```python
from build123d import *

# Parameters (mm, degrees)
SKETCH1_R           = 10
BOSS_EXTRUDE1_DEPTH = 15
CUT_EXTRUDE1_DEPTH  = 16
CUT_EXTRUDE2_DEPTH  = 10


with BuildPart() as part:
    # Sketch1 → Boss-Extrude1 (new body)
    with BuildSketch(Plane.XY):
        Circle(SKETCH1_R)
    extrude(amount=BOSS_EXTRUDE1_DEPTH)

    # Sketch2 → Cut-Extrude1 (cut, through all)
    with BuildSketch(Plane.XY.offset(15)):
        with BuildLine():
            Line((0, 0), (10, 0))
            ThreePointArc((10, 0), (7.071067812, -7.071067812), (0, -10))
            Line((0, -10), (0, 0))
        make_face()
    extrude(amount=-CUT_EXTRUDE1_DEPTH, mode=Mode.SUBTRACT)

    # Sketch5 → Cut-Extrude2 (cut)
    with BuildSketch(Plane(origin=(10, 0, 0), x_dir=(0, 0, -1), z_dir=(1, 0, 0))):
        Polygon((0, 0), (0, 10), (-15, 10), align=None)
    extrude(amount=-CUT_EXTRUDE2_DEPTH, mode=Mode.SUBTRACT)


solid = part.part
```
Check sheet for the modelled part. Datum: model origin and axes. Units: mm. A direction names the side the tool comes from. Coordinates: 2 decimals unless noted, no trailing zeros. Loops run counter-clockwise (first coordinate to the right, second up) from the corner with the lowest first, then second, coordinate; pieces in that order, holes last.
1) Sectioned sample at A-A (y = 8). Record the boundary of the cut face in (x, z).
2) Gauge pin test, flat ends, axial feed: pin 1 (5 mm diameter, centred on x = 8, z = 12, fed in from +Y); pin 2 (3 mm diameter, centred on y = 6.5, z = 4, fed in from -X); pin 3 (2 mm diameter, centred on y = -2.5, z = 8, fed in from -X). Record the tip position at first contact, or that the pin passes through.
3) Access from +Z, -Z, +X, -X, +Y, -Y to the whole of each face (thin tool, end or side, straight path). Record for faces 1 (the face through (5, 0, 8)), 2 (the face through (4, 4, 6)), 3 (the face through (-0.14, 0.14, 15)).
4) Sectioned sample at D-D (y = -7.25). Record the boundary of the cut face in (x, z).
5) Material ranges on probe 1 along X at (y, z) = (0.25, 5.75); probe 2 along Y at (x, z) = (8.25, 4.5); probe 3 along Y at (x, z) = (-3.25, 3.75), recorded low to high.
6) Sectioned sample at C-C (z = 8.75). Record the boundary of the cut face in (x, y), and give its area (3 significant figures).
7) Sectioned sample at B-B (x = -8). Record the boundary of the cut face in (y, z).
Check sheet entries:
1. outline: (-6, 0) - (0, 0) - (0, 12) - (6, 12) - (6, 15) - (-6, 15) - close
2. pin 1: stops at y = 8.32
2. pin 2: stops at x = -8.66
2. pin 3: stops at x = -9.89
3. face 1: +Z, -Z, +X, -Y
3. face 2: -Z, +X, +Y
3. face 3: +Z, +X, -X, +Y, -Y
4. outline: (-6.89, 0) - (0, 0) - (0, 15) - (-6.89, 15) - close
5. probe 1: x = -10 to 10
5. probe 2: y = 0 to 3
5. probe 3: y = -9.46 to 9.46
6. outline: (0, -10) - (0, 0) - (10, 0) arc R10 ccw to (8.12, 5.83) - (0, 5.83) - (0, 10) arc R10 ccw to start
6. area: 212 mm2
7. outline: (-6, 0) - (6, 0) - (6, 15) - (-6, 15) - close
